Autodesk Inventor part; units mm, degrees
ref_plane "YZ Plane" through (0, 0, 0) normal (1, 0, 0) x (0, 1, 0)
ref_plane "XZ Plane" through (0, 0, 0) normal (0, 1, 0) x (-1, 0, 0)
ref_plane "XY Plane" through (0, 0, 0) normal (0, 0, 1) x (1, 0, 0)
sketch "Skizze3" plane through (0, 0, 0) normal (1, 0, 0) x (0, 1, 0)
  line L0 (9.15, 0) -> (0, 0)
  line L1 (1.6, 5.55) -> (2.7, 5.55)
  line L2 (2.7, 5.55) -> (2.7, 2)
  line L3 (2.7, 2) -> (0, 2)
  line L4 (0, 2) -> (0, 7)
  line L5 (0, 7) -> (1.6, 7)
  line L6 (1.6, 7) -> (1.6, 5.55)
  dimension "d17" = 4
  dimension "d18" = 11.1
  dimension "d24" = 14
  dimension "d69" = 1.6
  dimension "d75" = 1.1
sketch "Skizze3 outline for Umdrehung1" plane through (0, 0, 0) normal (1, 0, 0) x (0, 1, 0)
  line L0 (1.6, 7) -> (0, 7)
  line L1 (1.6, 5.55) -> (1.6, 7)
  line L2 (2.7, 5.55) -> (1.6, 5.55)
  line L3 (2.7, 2) -> (2.7, 5.55)
  line L4 (0, 2) -> (2.7, 2)
  line L5 (0, 7) -> (0, 2)
revolve "Umdrehung1" add sketch "Skizze3 outline for Umdrehung1" angle 360 about axis through (0, 9.15, 0) along (0, -1, 0)
sketch "Skizze8" plane through (0, 2.7, 0) normal (0, 1, 0) x (1, 0, 0)
  circle A0 centre (0, 0) radius 5.55
  arc A1 (0.760995, -4.975916) -> (1.898212, -5.215294) centre (1.52199, -4.181632) ccw
  arc A2 (0.760995, -4.975916) -> (-0.760995, -4.975916) centre (0, -5.7702) ccw
  arc A3 (-1.898212, -5.215294) -> (-0.760995, -4.975916) centre (-1.52199, -4.181632) ccw
  line L0 (0, 9.8) -> (0, -9.8) construction
  line L1 (-1.898212, -5.215294) -> (0, 0) construction
  dimension "d59" = 1.1
  dimension "d60" = 1.1
  dimension "d61" = 20
sketch "Skizze8 outline for Extrusion5" plane through (0, 2.7, 0) normal (0, 1, 0) x (1, 0, 0)
  arc A0 (0.760995, -4.975916) -> (-0.760995, -4.975916) centre (0, -5.7702) ccw
  arc A1 (1.898212, -5.215294) -> (0.760995, -4.975916) centre (1.52199, -4.181632) cw
  arc A2 (-1.898212, -5.215294) -> (1.898212, -5.215294) centre (0, 0) ccw
  arc A3 (-0.760995, -4.975916) -> (-1.898212, -5.215294) centre (-1.52199, -4.181632) cw
extrude "Extrusion5" cut sketch "Skizze8 outline for Extrusion5" against normal up to surface (1.1 mm away)
pattern_circular "Runde Anordnung2" count 9 over 360 about axis through (0, -10, 0) along (0, 1, 0) of "Extrusion5"
sketch "Skizze9" plane through (0, 2.7, 5.7702) normal (0, 1, 0) x (1, 0, 0)
  circle A0 centre (0, 5.7702) radius 3 construction
  line L0 (0, 15.5702) -> (0, -4.0298) construction
  circle A1 centre (0, 5.7702) radius 2
  line L1 (-1.443376, 3.2702) -> (-2.886751, 5.7702)
  line L2 (-2.886751, 5.7702) -> (-1.443376, 8.2702)
  line L3 (-1.443376, 8.2702) -> (1.443376, 8.2702)
  line L4 (1.443376, 8.2702) -> (2.886751, 5.7702)
  line L5 (2.886751, 5.7702) -> (1.443376, 3.2702)
  line L6 (1.443376, 3.2702) -> (-1.443376, 3.2702)
  circle A2 centre (0, 10.2202) radius 1 construction
  arc A3 (0.986762, 10.706307) -> (-0.986762, 10.706307) centre (0, 10.2202) ccw construction
  line L7 (1.443376, 3.2702) -> (0, 5.7702)
  line L8 (0, 5.7702) -> (-1.443376, 3.2702)
  line L9 (1, 4.038149) -> (1, 3.2702)
  line L10 (-1, 4.038149) -> (-1, 3.2702)
  line L11 (1.443376, 3.2702) -> (1.443376, 4.385763)
  line L12 (-1.443376, 3.2702) -> (-1.443376, 4.385763)
  point P0 (0, 7.7702)
  point P1 (0, 11.2202)
  point P2 (1, 4.038149)
  point P3 (-1, 4.038149)
  dimension "d92" = 2
  dimension "d70" = 6
  dimension "d74" = 4
  dimension "d89" = 0.5
  dimension "d90" = 5
  dimension "d91" = 4.45
sketch "Skizze9 outline for Extrusion6" plane through (0, 2.7, 5.7702) normal (0, 1, 0) x (1, 0, 0)
  circle A0 centre (0, 5.7702) radius 2
  line L0 (1.443376, 3.2702) -> (2.886751, 5.7702)
  line L1 (2.886751, 5.7702) -> (1.443376, 8.2702)
  line L2 (1.443376, 8.2702) -> (-1.443376, 8.2702)
  line L3 (-1.443376, 8.2702) -> (-2.886751, 5.7702)
  line L4 (-2.886751, 5.7702) -> (-1.443376, 3.2702)
  line L5 (-1.443376, 3.2702) -> (1.443376, 3.2702)
extrude "Extrusion6" add sketch "Skizze9 outline for Extrusion6" along normal blind 3.3
hole "Bohrung3" at (0, 2.7, -4.45) direction (0, -1, 0) diameter 1.567 end through all
pattern_circular "Runde Anordnung3" count 3 over 360 about axis through (0, -10, 0) along (0, 1, 0) of "Bohrung3", "Extrusion6"
properties part number "Encoder Klemmscheibe" material "Aluminium 6061"
Work out the finished part from the listing and answer in its coordinate system (mm). A direction names the side the tool comes from. Give positions to 0.01 mm unless a question says otherwise; leave off trailing zeros. Write each loop counter-clockwise with the first axis right and the second up, starting at its lowest first coordinate (ties: lowest second). Pieces come first, ordered by that corner, then holes. Notation, with made-up numbers: (51.25, 57.5) - (75.25, 57.5) arc R18 cw to (75.25, 75.5) - close; hole circle Ø10 at (3, -21.5). An arc over 180 degrees is marked (long way). One line per item, written item: value. Start each with the question number.
1. Find section D-D (y = 1.1). State how many separate pieces and enclosed holes the cut face has, then the cut area to 3 significant figures.
2. For a pull along Z with two mould halves and no side action, classify faces 1 (the flat face through (-2.155, 4.327, -1.267)), 2 (the cylindrical face through (3.077, 1.331, 2.123)), 3 (the flat face through (2.155, 4.327, 1.267)) as +Z half, -Z half, draft (parallel to the pull), parting line (faces both ways), or undercut.
3. Find section B-B (z = -4). Write down the section's boundary in (x, y).
4. Find section A-A (x = -0.5). Write down the section's boundary in (y, z).
5. Consider probe 1 along Z at (x, y) = (0, 0.3); probe 2 along Z at (x, y) = (0, 3.5); probe 3 along Y at (x, z) = (-5, -3.25). Determine where each line is inside the solid, lowest interval first.
6. For faces 4 (the flat face through (-3, 2.7, 1)), 5 (the flat face through (0, 4, -2.5)), 6 (the flat face through (2.175, 4.327, -1.233)), 7 (the flat face through (0, 4, 2.5)), determine the directions among +Z, -Z, +X, -X, +Y, -Y from which every point of the face is accessible in a straight line to the end or side of a thin tool.
7. Find section C-C (x = 5.25). Write down the section's boundary in (y, z), then the cut area to 3 significant figures.
8. Given pin 1 (3 mm diameter, centred on x = -5, z = -1.5, fed in from +Y); pin 2 (6.5 mm diameter, centred on x = 0, z = 0, fed in from +Y); pin 3 (2 mm diameter, centred on y = 5, z = -0.5, fed in from +X); pin 4 (1.5 mm diameter, centred on x = 3, y = 5, fed in from -Z), each flat-ended and moving along its own axis, determine where each tip first touches the part or whether it passes through.
Geometry results:
1. separate pieces: 1
1. enclosed holes: 4
1. area: 136 mm2
2. face 1: -Z half
2. face 2: undercut
2. face 3: +Z half
3. outline: (-5.74, 0) - (-0.64, 0) - (-0.64, 2.7) - (-3.79, 2.7) - (-3.79, 1.6) - (-5.74, 1.6) - close; (0.64, 0) - (5.74, 0) - (5.74, 1.6) - (3.79, 1.6) - (3.79, 2.7) - (0.64, 2.7) - close
4. outline: (0, -6.98) - (1.6, -6.98) - (1.6, -5.43) - (2.7, -5.43) - (2.7, -5.05) - (0, -5.05) - close; (0, -3.85) - (2.7, -3.85) - (2.7, -2.5) - (6, -2.5) - (6, -1.94) - (0, -1.94) - close; (0, 1.94) - (6, 1.94) - (6, 2.5) - (2.7, 2.5) - (2.7, 4.79) - (1.6, 4.79) - (1.6, 6.98) - (0, 6.98) - close
5. probe 1: -7 to -5.23, -3.67 to -2, 2 to 7
5. probe 2: -2.5 to -2, 2 to 2.5
5. probe 3: 0 to 1.6
6. face 4: +Y
6. face 5: -Z, +X, -X, +Y
6. face 6: -Z, +X, +Y
6. face 7: +Z, +X, -X, +Y
7. outline: (0, -4.63) - (1.6, -4.63) - (1.6, -1.45) - (2.7, -1.45) - (2.7, -0.1) - (1.6, -0.1) - (1.6, 4.63) - (0, 4.63) - close
7. area: 16.3 mm2
8. pin 1: y = 2.7
8. pin 2: y = 6
8. pin 3: x = 2.89
8. pin 4: z = -1.1
